Autodesk Inventor part; units mm, degrees
ref_plane "YZ Plane" through (0, 0, 0) normal (1, 0, 0) x (0, 1, 0)
ref_plane "XZ Plane" through (0, 0, 0) normal (0, 1, 0) x (-1, 0, 0)
ref_plane "XY Plane" through (0, 0, 0) normal (0, 0, 1) x (1, 0, 0)
sketch "Sketch1" plane through (0, 0, 0) normal (0, 1, 0) x (-1, 0, 0)
  circle A0 centre (0, 0) radius 10
  dimension "d0" = 20
extrude "Extrusion1" add sketch "Sketch1" along normal mid plane 46
sketch "Sketch2" plane through (0, 23, 0) normal (0, 1, 0) x (1, 0, 0)
  circle A0 centre (0, 0) radius 10
hole "Hole1" at (0, 23, 0) direction (0, -1, 0) diameter 6 depth 10
sketch "Sketch3" plane through (0, -23, 0) normal (0, -1, 0) x (1, 0, 0)
  circle A0 centre (0, 0) radius 10
hole "Hole2" at (0, -23, 0) direction (0, 1, 0) diameter 6 depth 10
properties part number "Pneumatics Connector" material "Stainless Steel"
Geometry: final body of the model. Coordinates: model frame, mm. A direction names the side the tool comes from. Give positions to 0.01 mm unless a question says otherwise; leave off trailing zeros. Write each loop counter-clockwise with the first axis right and the second up, starting at its lowest first coordinate (ties: lowest second). Pieces come first, ordered by that corner, then holes. Notation, with made-up numbers: M 0.25,55 L 9.25,55 A12 cw 9.25,73 Z; hole C 66.25,37 d6. An arc over 180 degrees is marked long. Answer in a Markdown table with one row per item. Add a question column.
(1) Section D-D on y = -4. Return loops of the section in (x, z), and give its area (3 significant figures).
(2) Section A-A on y = -19. Return loops of the section in (x, z), and give its area (3 significant figures).
(3) Section B-B on x = 0. Return loops of the section in (y, z), and give its area (3 significant figures).
(4) Mould query, pull axis Z, two halves, no side actions, for faces 1 (the cylindrical face through (0, 18, -3)), 2 (the cylindrical face through (2.17, 0.32, -9.76)), 3 (the flat face through (-2.1, 23, 2.4)). Classes: +Z half, -Z half, draft (parallel to the pull), parting line (faces both ways), or undercut.
(5) Ray query, line 1 (Z direction, x = 0, y = -17); line 2 (Y direction, x = -0.75, z = 2); line 3 (Z direction, x = 4, y = 2.5). Return the intervals inside material, ascending.
(6) First-contact query: pin 1 (5.5 mm diameter, centred on x = 0, z = 0, fed in from +Y); pin 2 (1.8 mm diameter, centred on x = -1, z = -0.5, fed in from -Y); pin 3 (6 mm diameter, centred on y = 5, z = -7.5, fed in from -X). Flat tips, straight axial feed; report the tip coordinate or a pass-through.
(7) Section C-C on z = 0. Return loops of the section in (x, y).
(8) Reachability of faces 4 (the cylindrical face through (0, -18, 3)), 5 (the flat face through (0, 13, 0)), 6 (the flat face through (-2.1, -23, 2.4)) from +Z, -Z, +X, -X, +Y, -Y: full face, straight path, thin tool, end or side. Return the list, or none.
Result set:
| question | item | result |
|---|---|---|
| 1 | outline | C 0,0 d20 |
| 1 | area | 314 mm^2 |
| 2 | outline | C 0,0 d20; hole C 0,0 d6 |
| 2 | area | 286 mm^2 |
| 3 | outline | M -23,-10 L 23,-10 L 23,-3 L 13,-3 L 13,3 L 23,3 L 23,10 L -23,10 L -23,3 L -13,3 L -13,-3 L -23,-3 Z |
| 3 | area | 800 mm^2 |
| 4 | face 1 | undercut |
| 4 | face 2 | parting line |
| 4 | face 3 | draft |
| 5 | line 1 | z = -10 to -3, 3 to 10 |
| 5 | line 2 | y = -13 to 13 |
| 5 | line 3 | z = -9.17 to 9.17 |
| 6 | pin 1 | stops at y = 13 |
| 6 | pin 2 | stops at y = -13 |
| 6 | pin 3 | stops at x = -8.93 |
| 7 | outline | M -10,-23 L -3,-23 L -3,-13 L 3,-13 L 3,-23 L 10,-23 L 10,23 L 3,23 L 3,13 L -3,13 L -3,23 L -10,23 Z |
| 8 | face 4 | -Y |
| 8 | face 5 | +Y |
| 8 | face 6 | +Z, -Z, +X, -X, -Y |
